Check sheet for the modelled part. Datum: model origin and axes. Units: mm. A direction names the side the tool comes from. Give positions to 0.01 mm unless a question says otherwise; leave off trailing zeros. Loops run counter-clockwise (first coordinate to the right, second up) from the corner with the lowest first, then second, coordinate; pieces in that order, holes last.
```python
from build123d import *

# Parameters (mm, degrees)
SKETCH2_W           = 218
SKETCH2_H           = 30
BOSS_EXTRUDE1_DEPTH = 5
FILLET1_R           = 20
SKETCH3_R           = 10
CUT_EXTRUDE1_DEPTH  = 2
CHAMFER1_SIZE       = 3
SKETCH6_R           = 5
CUT_EXTRUDE2_DEPTH  = 119.749210232
BOSS_EXTRUDE2_DEPTH = 20
SKETCH8_W           = 30
SKETCH8_H           = 21.4
BOSS_EXTRUDE4_DEPTH = 3
SKETCH9_W           = 30
SKETCH9_H           = 21.4
CUT_EXTRUDE3_DEPTH  = 3
CUT_EXTRUDE4_DEPTH  = 40
FILLET2_R           = 10
CUT_EXTRUDE5_DEPTH  = 40
FILLET3_R           = 10


with BuildPart() as part:
    # Sketch2 → Boss-Extrude1 (new, symmetric)
    with BuildSketch(Plane.XY):
        Rectangle(SKETCH2_W, SKETCH2_H)
    extrude(amount=BOSS_EXTRUDE1_DEPTH, both=True)

    # Fillet1
    fillet1_edges = [part.edges().sort_by_distance(p)[0] for p in [
        (109, -15, 0),
        (-109, -15, 0),
    ]]
    fillet(fillet1_edges, radius=FILLET1_R)

    # Sketch3 → Cut-Extrude1 (cut, symmetric)
    with BuildSketch(Plane.XY.offset(5)):
        with Locations((-91, 2)):
            Circle(SKETCH3_R)
        with Locations((-31, 2)):
            Circle(SKETCH3_R)
    extrude(amount=CUT_EXTRUDE1_DEPTH, both=True, mode=Mode.SUBTRACT)

    # Chamfer1
    # the kernel refuses this chamfer: 3 mm, written as the material it takes off along each edge
    with BuildSketch(Plane(origin=(-31, 2, 5), x_dir=(1, 0, 0), z_dir=(0, -1, 0))) as chamfer1_piece_1_section:
        Polygon((10 + CHAMFER1_SIZE, 0), (10, -CHAMFER1_SIZE), (10, 0), align=None)
    chamfer1_piece_1 = revolve(axis=Axis((-31, 2, 5), (0, 0, 1)), mode=Mode.PRIVATE)
    chamfer1_piece_1 = split(chamfer1_piece_1, bisect_by=Plane(origin=(-42.994962735, 2, 3), z_dir=(0, 0, 1)), keep=Keep.TOP, mode=Mode.PRIVATE)
    add(chamfer1_piece_1, mode=Mode.SUBTRACT)
    with BuildSketch(Plane(origin=(-91, 2, 5), x_dir=(1, 0, 0), z_dir=(0, -1, 0))) as chamfer1_piece_2_section:
        Polygon((10 + CHAMFER1_SIZE, 0), (10, -CHAMFER1_SIZE), (10, 0), align=None)
    chamfer1_piece_2 = revolve(axis=Axis((-91, 2, 5), (0, 0, 1)), mode=Mode.PRIVATE)
    chamfer1_piece_2 = split(chamfer1_piece_2, bisect_by=Plane(origin=(-102.994962728, 2, 3), z_dir=(0, 0, 1)), keep=Keep.TOP, mode=Mode.PRIVATE)
    add(chamfer1_piece_2, mode=Mode.SUBTRACT)

    # Sketch5 → Revolve1 (revolve)
    with BuildSketch(Plane(origin=(-61.85, 0, 0), x_dir=(0, 0, -1), z_dir=(1, 0, 0)), mode=Mode.PRIVATE) as revolve1_sk:
        Polygon((-20.498711306, 18.495190528), (-24.248711306, 12), (10.392304845, -8), (14.142304845, -1.504809472), align=None)
    revolve(revolve1_sk.sketch.rotate(Axis((-61.85, 12, 24.248711306), (0, -0.4999999999999977, -0.86602540378444)), 180), axis=Axis((-61.85, 12, 24.248711306), (0, -0.4999999999999977, -0.86602540378444)))

    # Sketch6 → Cut-Extrude2 (cut, through all)
    with BuildSketch(Plane(origin=(0, 13.5, 23.382685902), x_dir=(1, 0, 0), z_dir=(0, 0.4999999999999978, 0.86602540378444))):
        with Locations(Location((-61.85, -1.732050808, 0), (0, 0, 270))):
            Circle(SKETCH6_R)
    extrude(amount=-CUT_EXTRUDE2_DEPTH, mode=Mode.SUBTRACT)

    # Sketch7 → Boss-Extrude2 (add, symmetric)
    with BuildSketch(Plane(origin=(0, 0, 0), x_dir=(0, 0, -1), z_dir=(1, 0, 0))):
        Polygon((5, -15), (-5, -15), (-33.867513459, -65), (-91.641016151, -65), (-91.641016151, -75), (-29.641016151, -75), align=None)
    extrude(amount=BOSS_EXTRUDE2_DEPTH, both=True)

    # Sketch8 → Boss-Extrude4 (add)
    with BuildSketch(Plane(origin=(0, -1.584936491, -2.745190528), x_dir=(1, 0, 0), z_dir=(0, 0.49999999999999756, 0.86602540378444))):
        with Locations((0, -31.190381057)):
            Rectangle(SKETCH8_W, SKETCH8_H)
    extrude(amount=BOSS_EXTRUDE4_DEPTH)

    # Sketch9 → Cut-Extrude3 (cut)
    with BuildSketch(Plane(origin=(0, -1.584936491, -2.745190528), x_dir=(1, 0, 0), z_dir=(0, 0.49999999999999756, 0.86602540378444))):
        with Locations((0, -57.525407976)):
            Rectangle(SKETCH9_W, SKETCH9_H)
    extrude(amount=-CUT_EXTRUDE3_DEPTH, mode=Mode.SUBTRACT)

    # Sketch10 → Revolve2 (revolve)
    with BuildSketch(Plane(origin=(0, 0, 0), x_dir=(0, 0, -1), z_dir=(1, 0, 0)), mode=Mode.PRIVATE) as revolve2_sk:
        with BuildLine():
            Line((-61.641016151, -23.080849404), (-61.641016151, -85))
            Line((-61.641016151, -85), (-54.141016151, -85))
            Line((-54.141016151, -85), (-54.141016151, -75))
            Line((-54.141016151, -75), (-56.641016151, -75))
            Line((-56.641016151, -75), (-56.641016151, -63))
            ThreePointArc((-56.641016151, -63), (-57.519695808, -60.878679656), (-59.641016151, -60))
            Line((-59.641016151, -60), (-59.641016151, -36.590975833))
            ThreePointArc((-59.641016151, -36.590975833), (-54.904038671, -28.986627083), (-61.641016151, -23.080849404))
        make_face()
    revolve(revolve2_sk.sketch.rotate(Axis((0, -23.080849404, 61.641016151), (0, -1, 0)), 180), axis=Axis((0, -23.080849404, 61.641016151), (0, -1, 0)))

    # Sketch11 → Cut-Extrude4 (cut)
    with BuildSketch(Plane(origin=(0, 15, 0), x_dir=(1, 0, 0), z_dir=(0, 1, 0))):
        Polygon((-109, 5), (-109, -5), (-105.52, 5), align=None)
    extrude(amount=-CUT_EXTRUDE4_DEPTH, mode=Mode.SUBTRACT)

    # Fillet2
    fillet2_edges = [part.edges().sort_by_distance(p)[0] for p in [
        (-107.26, 15, 0),
    ]]
    fillet(fillet2_edges, radius=FILLET2_R)

    # Sketch13 → Cut-Extrude5 (cut)
    with BuildSketch(Plane(origin=(0, 15, 0), x_dir=(1, 0, 0), z_dir=(0, 1, 0))):
        Polygon((109, 5), (109, -5), (105.52, 5), align=None)
    extrude(amount=-CUT_EXTRUDE5_DEPTH, mode=Mode.SUBTRACT)

    # Fillet3
    fillet3_edges = [part.edges().sort_by_distance(p)[0] for p in [
        (107.26, 15, 0),
    ]]
    fillet(fillet3_edges, radius=FILLET3_R)


solid = part.part
```
(1) Section check A-A on z = 84. Record the boundary of the cut face in (x, y).
(2) Release check for a two-part mould opening along Z. For faces 1 (the face through (-64.1, 0.73, 19.04)), 2 (the face through (103.816, 12.148, -0.748)), 3 (the face through (-2.253, -79.93, 68.795)) record: pulls with the +Z half, pulls with the -Z half, needs draft (parallel to the pull), parting line crosses it, or undercut.
(3) Material ranges on line 1 (Y direction, x = -19.5, z = 54); line 2 (Z direction, x = 92, y = 2.5); line 3 (X direction, y = 6, z = 25), recorded low to high.
(4) Access from +Z, -Z, +X, -X, +Y, -Y to the whole of each face (thin tool, end or side, straight path). Record for faces 4 (the face through (54, -15, 0)), 5 (the face through (-55, -15, 0)), 6 (the face through (-91, 2, 3)), 7 (the face through (5, -75, 68)), 8 (the face through (0, -70, 91.641)).
(5) Section check B-B on x = -47.5. Record the boundary of the cut face in (y, z).
(6) Gauge pin test, flat ends, axial feed: pin 1 Ø5 at (x, z) = (60.5, -1.5) entering from -Y; pin 2 Ø4 at (x, y) = (-82.5, -10) entering from -Z; pin 3 Ø1.5 at (y, z) = (-71, 64.5) entering from +X; pin 4 Ø12 at (y, z) = (-48.5, 4) entering from +X. Record the tip position at first contact, or that the pin passes through.
Computed values:
1. outline: (-20, -75) - (20, -75) - (20, -65) - (-20, -65) - close
2. face 1: undercut
2. face 2: pulls with the -Z half
2. face 3: parting line crosses it
3. line 1: y = -75 to -65
3. line 2: z = -5 to 5
3. line 3: x = -66.87 to -56.83
4. face 4: +Z, -Z, +X, -Y
4. face 5: +Z, -Z, -X, -Y
4. face 6: +Z
4. face 7: -Y
4. face 8: +Z, +X, -X, +Y, -Y
5. outline: (-15, -5) - (15, -5) - (15, 5) - (-15, 5) - close
6. pin 1: stops at y = -15
6. pin 2: stops at z = -5
6. pin 3: stops at x = 20
6. pin 4: passes through
